Geometry check sheet. Reference: drawing and pictorial views, mm from the part's lowest x, y, z. A direction names the side the tool comes from. Give positions to 0.01 mm unless a question says otherwise; leave off trailing zeros. Order: outer loops, then holes, each group sorted by start corner. A loop starts at its lowest first (then second) coordinate and runs counter-clockwise, first axis right, second up. Notation, with made-up numbers: M 71,75.5 L 125,75.5 A12 ccw 125,93.5 Z; hole C 36,-0.75 d7. An arc over 180 degrees is marked long. Answer as CSV lines item,"result".
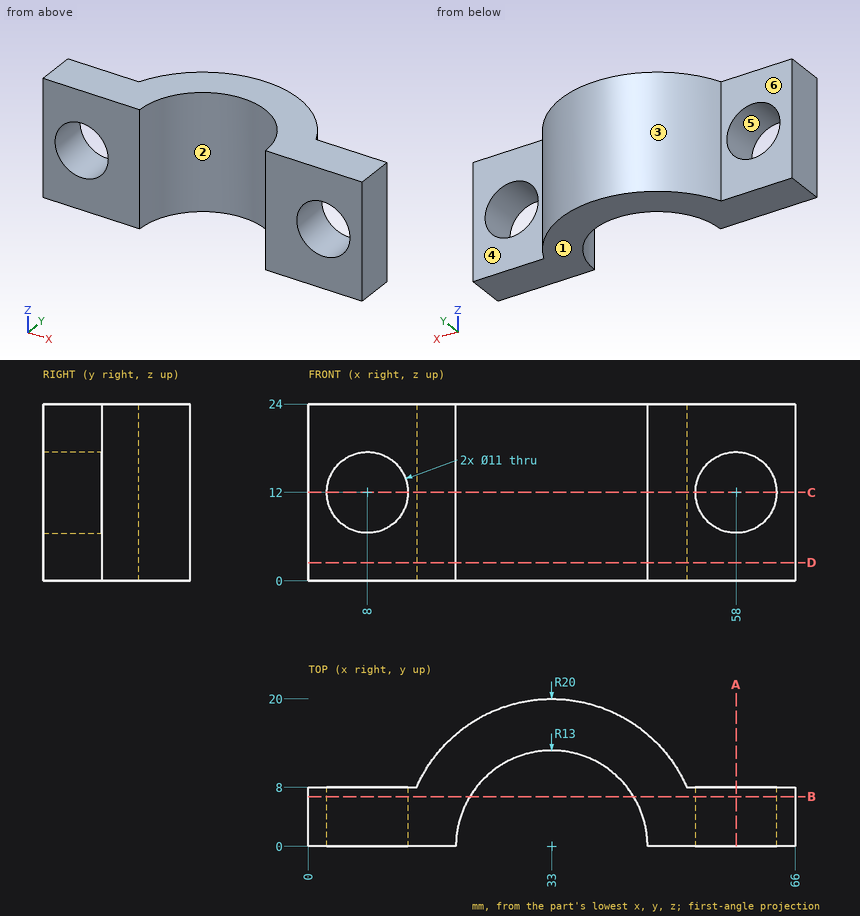
(1) Section check D-D on z = 2.5. Enter the section's corners in (x, y).
The answers:
outline,"M 0,0 L 20,0 A13 cw 46,0 L 66,0 L 66,8 L 51.33,8 A20 ccw 14.67,8 L 0,8 Z"
(2) Section check C-C on z = 12. Enter the section's corners in (x, y).
The answers:
outline,"M 0,0 L 2.5,0 L 2.5,8 L 0,8 Z; M 13.5,0 L 20,0 A13 cw 46,0 L 52.5,0 L 52.5,8 L 51.33,8 A20 ccw 14.67,8 L 13.5,8 Z; M 63.5,0 L 66,0 L 66,8 L 63.5,8 Z"
(3) Tool access check on the marked faces 4, 5 and 6. Record the directions out of +Z, -Z, +X, -X, +Y, -Y that give a thin tool (end or side, any length) a straight path to the whole face; none if there is none.
The answers:
face 4,"+Z, -Z, +X, +Y"
face 5,"+Y, -Y"
face 6,"+Z, -Z, -X, +Y"
(4) Section check B-B on y = 6.75. Enter the section's corners in (x, z).
The answers:
outline,"M 0,0 L 21.89,0 L 21.89,24 L 0,24 Z; M 44.11,0 L 66,0 L 66,24 L 44.11,24 Z; hole C 8,12 d11; hole C 58,12 d11"
(5) Draft check along X on the marked faces 1, 2 and 3. Enter one of: +X half, -X half, draft (parallel to the pull), parting line (faces both ways), or undercut.
The answers:
face 1,"draft"
face 2,"undercut"
face 3,"parting line"
(6) Material ranges on line 1 (Z direction, x = 8, y = 5); line 2 (X direction, y = 2, z = 13.5); line 3 (X direction, y = 4.25, z = 11), recorded low to high.
The answers:
line 1,"z = 0 to 6.5, 17.5 to 24"
line 2,"x = 0 to 2.71, 13.29 to 20.15, 45.85 to 52.71, 63.29 to 66"
line 3,"x = 0 to 2.59, 13.41 to 20.71, 45.29 to 52.59, 63.41 to 66"
(7) Gauge pin test, flat ends, axial feed: P1, Ø11.5, axis at x = 10.5, z = 13, coming from the +Y side; P2, Ø5, axis at x = 50.5, z = 17.5, coming from the +Y side; P3, Ø6.5, axis at x = 58, z = 12, coming from the -Y side; P4, Ø4.5, axis at x = 58.5, z = 17, coming from the +Y side. Record the tip position at first contact, or that the pin passes through.
The answers:
P1,"stops at y = 10.93"
P2,"stops at y = 13.23"
P3,"passes through"
P4,"stops at y = 8"
(8) Section check A-A on x = 58. Enter the section's corners in (y, z).
The answers:
outline,"M 0,0 L 8,0 L 8,6.5 L 0,6.5 Z; M 0,17.5 L 8,17.5 L 8,24 L 0,24 Z"
